Read the model definition and answer for the solid it produces. Units are mm, in the model's axes. A direction names the side the tool comes from. Give positions to 0.01 mm unless a question says otherwise; leave off trailing zeros. Order: outer loops, then holes, each group sorted by start corner. A loop starts at its lowest first (then second) coordinate and runs counter-clockwise, first axis right, second up. Notation, with made-up numbers: (60, 8) - (119, 8) arc R12 ccw to (119, 12) - close; hole circle Ø8 at (-40, 38.5). An arc over 180 degrees is marked (long way). Return JSON: item names as keys, results as strings.
```python
from build123d import *

# Parameters (mm, degrees)
F1_DEPTH  = 76.2
F2_R      = 19.05
F3_DEPTH  = 12.7
F4_R      = 12.7
F5_DEPTH  = 12.7
F6_R      = 12.7
F7_DEPTH  = 63.5
F8_R      = 19.05
F9_DEPTH  = 12.7
F10_R     = 12.7
F11_DEPTH = 15.875


with BuildPart() as f1:
    # F0 (on Front) → F1 (new body)
    with BuildSketch(Plane.XZ):
        with BuildLine():
            Line((0, 76.2), (0, 0))
            Line((0, 0), (177.8, 0))
            Line((177.8, 0), (177.8, 28.575))
            Line((177.8, 28.575), (82.651526, 28.575))
            Line((82.651526, 28.575), (82.651526, 76.2))
            ThreePointArc((82.651526, 76.2), (41.325763, 117.525763), (0, 76.2))
        make_face()
    extrude(amount=F1_DEPTH)

    # F2 (on face) → F3 (cut)
    with BuildSketch(Plane.XZ.offset(76.2)):
        with Locations((41.325763, 76.2)):
            Circle(F2_R)
    extrude(amount=-F3_DEPTH, mode=Mode.SUBTRACT)

    # F4 (on face) → F5 (cut, through all)
    with BuildSketch(Plane.XZ.offset(76.2)):
        with Locations((41.325763, 76.2)):
            Circle(F4_R)
    extrude(amount=-F5_DEPTH, mode=Mode.SUBTRACT)

    # F6 (on face) → F7 (cut, through all)
    with BuildSketch(Plane.XZ.offset(63.5)):
        with Locations((41.325763, 76.2)):
            Circle(F6_R)
    extrude(amount=-F7_DEPTH, mode=Mode.SUBTRACT)

    # F8 (on face) → F9 (cut)
    with BuildSketch(Plane.XY.offset(28.575)):
        with Locations((139.7, -38.1)):
            Circle(F8_R)
    extrude(amount=-F9_DEPTH, mode=Mode.SUBTRACT)

    # F10 (on face) → F11 (cut, through all)
    with BuildSketch(Plane.XY.offset(15.875)):
        with Locations((139.7, -38.1)):
            Circle(F10_R)
    extrude(amount=-F11_DEPTH, mode=Mode.SUBTRACT)


solid = f1.part
```
Q1. A cutting plane is placed at A-A (y = -38.1). Write down the section's boundary in (x, z) (3 decimals), and give its area (3 significant figures).
Values:
{"outline": "(0, 0) - (127, 0) - (127, 15.875) - (120.65, 15.875) - (120.65, 28.575) - (82.652, 28.575) - (82.652, 76.2) arc R41.326 ccw to (0, 76.2) - close; (152.4, 0) - (177.8, 0) - (177.8, 28.575) - (158.75, 28.575) - (158.75, 15.875) - (152.4, 15.875) - close; hole circle Ø25.4 at (41.326, 76.2)", "area": "10,300 mm²"}
Q2. A cutting plane is placed at B-B (x = 139.7). Write down the section's boundary in (y, z) (3 decimals).
Values:
{"outline": "(-76.2, 0) - (-50.8, 0) - (-50.8, 15.875) - (-57.15, 15.875) - (-57.15, 28.575) - (-76.2, 28.575) - close; (-25.4, 0) - (0, 0) - (0, 28.575) - (-19.05, 28.575) - (-19.05, 15.875) - (-25.4, 15.875) - close"}
Q3. Given pin 1 (10 mm diameter, centred on x = 127, y = -27, fed in from +Z) (3 decimals); pin 2 (19 mm diameter, centred on x = 35, z = 74, fed in from -Y); pin 3 (24 mm diameter, centred on y = -34, z = 47, fed in from +X); pin 4 (12 mm diameter, centred on x = 64, z = 78.5, fed in from +Y), each flat-ended and moving along its own axis, determine where each tip first touches the part or whether it passes through.
Values:
{"pin 1": "stops at z = 28.575", "pin 2": "stops at y = -63.5", "pin 3": "stops at x = 82.65", "pin 4": "stops at y = 0"}
Q4. Consider L1, parallel to X at y = -38, z = 22; L2, parallel to Y at x = 139, z = 22; L3, parallel to X at y = -68, z = 76. Determine where each line is inside the solid, lowest interval first.
Values:
{"L1": "x = 0 to 120.65, 158.75 to 177.8", "L2": "y = -76.2 to -57.14, -19.06 to 0", "L3": "x = 0 to 22.28, 60.37 to 82.65"}
Q5. A cutting plane is placed at D-D (z = 86). Write down the section's boundary in (x, y), and give its area (3 significant figures).
Values:
{"outline": "(1.18, -76.2) - (24.99, -76.2) - (24.99, -63.5) - (33.25, -63.5) - (33.25, 0) - (1.18, 0) - close; (49.4, -63.5) - (57.66, -63.5) - (57.66, -76.2) - (81.47, -76.2) - (81.47, 0) - (49.4, 0) - close", "area": "4,680 mm²"}
Q6. Determine the mould class of faces 6 (the flat face through (68, -76.2, 47)), 7 (the cylindrical face through (42.234, -37.567, 117.516)), 8 (the flat face through (54, -63.5, 72)) for opening direction X: released by +X, released by -X, zero draft, split by the parting line, or undercut.
Values:
{"face 6": "zero draft", "face 7": "split by the parting line", "face 8": "undercut"}
Q7. For faces 1 (the cylindrical face through (151.432, -42.964, 8.049)), 2 (the flat face through (82.652, -38, 52)), 3 (the flat face through (152, -42, 15.875)), 4 (the cylindrical face through (38.85, -69.94, 95.09)), 5 (the flat face through (88, -38, 0)), determine the directions among +Z, -Z, +X, -X, +Y, -Y from which every point of the face is accessible in a straight line to the end or side of a thin tool.
Values:
{"face 1": "+Z, -Z", "face 2": "+Z, +X, +Y, -Y", "face 3": "+Z", "face 4": "-Y", "face 5": "-Z, +X, -X, +Y, -Y"}
Q8. A cutting plane is placed at C-C (y = -5.5). Write down the section's boundary in (x, z) (3 decimals), and give its area (3 significant figures).
Values:
{"outline": "(0, 0) - (177.8, 0) - (177.8, 28.575) - (82.652, 28.575) - (82.652, 76.2) arc R41.326 ccw to (0, 76.2) - close; hole circle Ø25.4 at (41.326, 76.2)", "area": "11,200 mm²"}
